Work out the finished part from the listing and answer in its coordinate system (mm). A direction names the side the tool comes from. Round coordinates to 2 decimals unless told otherwise and drop trailing zeros. Loops run counter-clockwise (first coordinate to the right, second up) from the corner with the lowest first, then second, coordinate; pieces in that order, holes last. Notation, with made-up numbers: (58, -18.75) - (65, -18.75) arc R24 cw to (65, 11.25) - close; hole circle Ø7 at (33, 47.25). An arc over 180 degrees is marked (long way). Return JSON: item names as keys, results as strings.
from build123d import *

# Parameters (mm, degrees)
SKETCH1_W           = 11.5
SKETCH1_H           = 7.8
BOSS_EXTRUDE1_DEPTH = 340
SKETCH2_W           = 0.835250229
SKETCH2_H           = 1.6
CUT_EXTRUDE1_DEPTH  = 341.070981561
SKETCH3_R           = 3
CUT_EXTRUDE2_DEPTH  = 4.7
SKETCH4_R           = 1.7
CUT_EXTRUDE3_DEPTH  = 341.081096946


with BuildPart() as part:
    # Sketch1 → Boss-Extrude1 (new body)
    with BuildSketch(Plane.XY):
        Rectangle(SKETCH1_W, SKETCH1_H)
    extrude(amount=BOSS_EXTRUDE1_DEPTH)

    # Sketch2 → Cut-Extrude1 (cut, through all)
    with BuildSketch(Plane.XY.offset(340)):
        with Locations((5.332374886, 1.7)):
            Rectangle(SKETCH2_W, SKETCH2_H)
        with Locations((-5.332374886, 1.7)):
            Rectangle(SKETCH2_W, SKETCH2_H)
    extrude(amount=-CUT_EXTRUDE1_DEPTH, mode=Mode.SUBTRACT)

    # Sketch3 → Cut-Extrude2 (cut)
    with BuildSketch(Plane(origin=(0, 3.9, 0), x_dir=(1, 0, 0), z_dir=(0, 1, 0))):
        with Locations(Location((0, -328.4, 0), (0, 0, 270))):
            Circle(SKETCH3_R)
        with Locations(Location((0, -303.4, 0), (0, 0, 270))):
            Circle(SKETCH3_R)
        with Locations(Location((0, -278.4, 0), (0, 0, 270))):
            Circle(SKETCH3_R)
        with Locations(Location((0, -253.4, 0), (0, 0, 270))):
            Circle(SKETCH3_R)
        with Locations(Location((0, -228.4, 0), (0, 0, 270))):
            Circle(SKETCH3_R)
        with Locations(Location((0, -203.4, 0), (0, 0, 270))):
            Circle(SKETCH3_R)
        with Locations(Location((0, -178.4, 0), (0, 0, 270))):
            Circle(SKETCH3_R)
        with Locations(Location((0, -153.4, 0), (0, 0, 270))):
            Circle(SKETCH3_R)
        with Locations(Location((0, -128.4, 0), (0, 0, 270))):
            Circle(SKETCH3_R)
        with Locations(Location((0, -103.4, 0), (0, 0, 270))):
            Circle(SKETCH3_R)
        with Locations(Location((0, -78.4, 0), (0, 0, 270))):
            Circle(SKETCH3_R)
        with Locations(Location((0, -53.4, 0), (0, 0, 270))):
            Circle(SKETCH3_R)
        with Locations(Location((0, -28.4, 0), (0, 0, 270))):
            Circle(SKETCH3_R)
        with Locations(Location((0, -3.4, 0), (0, 0, 270))):
            Circle(SKETCH3_R)
        with Locations((0, 21.6)):
            Circle(SKETCH3_R)
        with Locations((0, 46.6)):
            Circle(SKETCH3_R)
        with Locations((0, 71.6)):
            Circle(SKETCH3_R)
        with Locations((0, 96.6)):
            Circle(SKETCH3_R)
        with Locations((0, 121.6)):
            Circle(SKETCH3_R)
        with Locations((0, 146.6)):
            Circle(SKETCH3_R)
        with Locations((0, 171.6)):
            Circle(SKETCH3_R)
        with Locations((0, 196.6)):
            Circle(SKETCH3_R)
        with Locations((0, 221.6)):
            Circle(SKETCH3_R)
        with Locations((0, 246.6)):
            Circle(SKETCH3_R)
        with Locations((0, 271.6)):
            Circle(SKETCH3_R)
    extrude(amount=-CUT_EXTRUDE2_DEPTH, mode=Mode.SUBTRACT)

    # Sketch4 → Cut-Extrude3 (cut, through all)
    with BuildSketch(Plane(origin=(0, -0.8, 0), x_dir=(1, 0, 0), z_dir=(0, 1, 0))):
        with Locations(Location((0, -328.4, 0), (0, 0, 270))):
            Circle(SKETCH4_R)
        with Locations(Location((0, -303.4, 0), (0, 0, 270))):
            Circle(SKETCH4_R)
        with Locations(Location((0, -278.4, 0), (0, 0, 270))):
            Circle(SKETCH4_R)
        with Locations(Location((0, -253.4, 0), (0, 0, 270))):
            Circle(SKETCH4_R)
        with Locations(Location((0, -228.4, 0), (0, 0, 270))):
            Circle(SKETCH4_R)
        with Locations(Location((0, -203.4, 0), (0, 0, 270))):
            Circle(SKETCH4_R)
        with Locations(Location((0, -178.4, 0), (0, 0, 270))):
            Circle(SKETCH4_R)
        with Locations(Location((0, -153.4, 0), (0, 0, 270))):
            Circle(SKETCH4_R)
        with Locations(Location((0, -128.4, 0), (0, 0, 270))):
            Circle(SKETCH4_R)
        with Locations(Location((0, -103.4, 0), (0, 0, 270))):
            Circle(SKETCH4_R)
        with Locations(Location((0, -78.4, 0), (0, 0, 270))):
            Circle(SKETCH4_R)
        with Locations(Location((0, -53.4, 0), (0, 0, 270))):
            Circle(SKETCH4_R)
        with Locations(Location((0, -28.4, 0), (0, 0, 270))):
            Circle(SKETCH4_R)
        with Locations(Location((0, -3.4, 0), (0, 0, 270))):
            Circle(SKETCH4_R)
        with Locations((0, 21.6)):
            Circle(SKETCH4_R)
        with Locations((0, 46.6)):
            Circle(SKETCH4_R)
        with Locations((0, 71.6)):
            Circle(SKETCH4_R)
        with Locations((0, 96.6)):
            Circle(SKETCH4_R)
        with Locations((0, 121.6)):
            Circle(SKETCH4_R)
        with Locations((0, 146.6)):
            Circle(SKETCH4_R)
        with Locations((0, 171.6)):
            Circle(SKETCH4_R)
        with Locations((0, 196.6)):
            Circle(SKETCH4_R)
        with Locations((0, 221.6)):
            Circle(SKETCH4_R)
        with Locations((0, 246.6)):
            Circle(SKETCH4_R)
        with Locations((0, 271.6)):
            Circle(SKETCH4_R)
    extrude(amount=-CUT_EXTRUDE3_DEPTH, mode=Mode.SUBTRACT)


solid = part.part
1) A tool of negligible diameter and unlimited length cuts with its end or side. For faces 3 (the cylindrical face through (-1.8, 1.6, 101)), 4 (the flat face through (0, 0, 0)), from which of +Z, -Z, +X, -X, +Y, -Y can it reach the whole face along a straight path? Write none if from no direction.
Verdict:
{"face 3": "+Y", "face 4": "-Z, +X, -X, +Y, -Y"}
2) Flat-ended cylindrical pins translate along their axes: pin 1 (1.8 mm diameter, centred on x = 1, z = 228.5, fed in from +Y); pin 2 (1 mm diameter, centred on y = 1.5, z = 186.5, fed in from -X). Find the tip coordinate at first contact, or state that the pin passes through.
Verdict:
{"pin 1": "stops at y = -0.8", "pin 2": "stops at x = -4.91"}
3) Determine the mould class of faces 1 (the cylindrical face through (0.9, 1.58, 56.26)), 2 (the flat face through (0, 0, 340)) for opening direction X: pulls with the +X half, pulls with the -X half, needs draft (parallel to the pull), parting line crosses it, or undercut.
Verdict:
{"face 1": "undercut", "face 2": "needs draft"}
4) Find the intervals of material crossed by L1, parallel to X at y = 1.15, z = 328.4; L2, parallel to X at y = 1.25, z = 154; L3, parallel to X at y = 2, z = 143.5, in increasing order.
Verdict:
{"L1": "x = -4.91 to -3, 3 to 4.91", "L2": "x = -4.91 to -2.94, 2.94 to 4.91", "L3": "x = -4.91 to 4.91"}
5) Section A-A (z = 239) is taken. Give the vertices of the cut face in (x, y), and give its area (3 significant figures).
Verdict:
{"outline": "(-5.75, -3.9) - (5.75, -3.9) - (5.75, 0.9) - (4.91, 0.9) - (4.91, 2.5) - (5.75, 2.5) - (5.75, 3.9) - (-5.75, 3.9) - (-5.75, 2.5) - (-4.91, 2.5) - (-4.91, 0.9) - (-5.75, 0.9) - close", "area": "87.0 mm2"}
